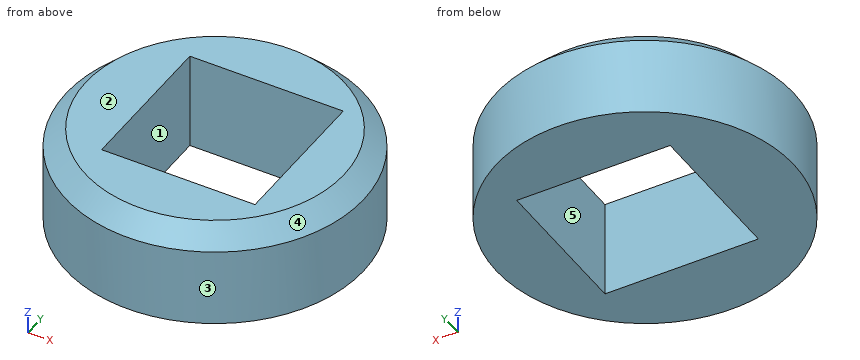
from build123d import *

# Parameters (mm, degrees)
F0_R     = 37.945444
F1_DEPTH = 25
F2_W     = 39.141135
F2_H     = 38.724022
F3_DEPTH = 25
F4_SIZE  = 5


with BuildPart() as f1:
    # F0 (on Top) → F1 (new body)
    with BuildSketch(Plane.XY):
        Circle(F0_R)
    extrude(amount=F1_DEPTH)

    # F2 (on face) → F3 (cut)
    with BuildSketch(Plane.XY.offset(25)):
        with Locations((1.78278, 0.198509)):
            Rectangle(F2_W, F2_H)
    extrude(amount=-F3_DEPTH, mode=Mode.SUBTRACT)

    # F4
    f4_edges = [f1.edges().sort_by_distance(p)[0] for p in [
        (-37.945444, 0, 25),
    ]]
    chamfer(f4_edges, length=F4_SIZE)


solid = f1.part
Could you check a few things on this model? Use its own coordinates, in mm. Face numbers are marked on the shaded views. A direction names the side the tool comes from. Give positions to 0.01 mm unless a question says otherwise; leave off trailing zeros. Order: outer loops, then holes, each group sorted by start corner. A loop starts at its lowest first (then second) coordinate and runs counter-clockwise, first axis right, second up. Notation, with made-up numbers: (29, -15) -> (81, -15) arc R18 cw to (81, -9) -> close; hole circle Ø1 at (7, -6). An arc over 180 degrees is marked (long way). Return JSON: item names as keys, results as strings.
1. Thinking about a two-plate mould opening in Y: for the marked faces 1, 2 and 3, which applies, pulls with the +Y half, pulls with the -Y half, needs draft (parallel to the pull), parting line crosses it, or undercut?
Answer list:
{"face 1": "undercut", "face 2": "needs draft", "face 3": "parting line crosses it"}
2. For pin 1 Ø7.5 at (y, z) = (2, 16.5) entering from +X; pin 2 Ø5 at (x, z) = (30, 20.5) entering from -Y; pin 3 Ø10 at (y, z) = (-22, 14) entering from -X; pin 4 Ø12.5 at (x, z) = (-1, 16) entering from -Y, each with a flat end and sliding along its axis, tell me the tip position at first contact or that it passes through.
Answer list:
{"pin 1": "stops at x = 37.95", "pin 2": "stops at y = -26.09", "pin 3": "stops at x = -33.92", "pin 4": "stops at y = -37.95"}
3. On a 3-axis mill with a long thin cutter (end or side, diameter ignored), from which of +Z, -Z, +X, -X, +Y, -Y can I reach the whole of each face in a straight line? I mean the marked faces 4 and 5. Say none if no direction works.
Answer list:
{"face 4": "+Z", "face 5": "+Z, -Z"}
4. I need wall thicknesses on line 1 (X direction, y = 0.5, z = 17.5); line 2 (X direction, y = -9, z = 3); line 3 (Y direction, x = 16, z = 9.5). Which ranges of each line are inside material? Lowest first, please. Write a range as from..to.
Answer list:
{"line 1": "x = -37.94..-17.79, 21.35..37.94", "line 2": "x = -36.86..-17.79, 21.35..36.86", "line 3": "y = -34.41..-19.16, 19.56..34.41"}
5. Imagine slicing it at B-B on y = 0. List the corners of the cut face in (x, z) for me.
Answer list:
{"outline": "(-37.95, 0) -> (-17.79, 0) -> (-17.79, 25) -> (-32.95, 25) -> (-37.95, 20) -> close; (21.35, 0) -> (37.95, 0) -> (37.95, 20) -> (32.95, 25) -> (21.35, 25) -> close"}
6. Imagine slicing it at A-A on x = 0. List the corners of the cut face in (y, z) for me.
Answer list:
{"outline": "(-37.95, 0) -> (-19.16, 0) -> (-19.16, 25) -> (-32.95, 25) -> (-37.95, 20) -> close; (19.56, 0) -> (37.95, 0) -> (37.95, 20) -> (32.95, 25) -> (19.56, 25) -> close"}
7. Imagine slicing it at C-C on z = 7.5. List the corners of the cut face in (x, y) for me.
Answer list:
{"outline": "circle Ø75.89 at (0, 0); hole (-17.79, -19.16) -> (21.35, -19.16) -> (21.35, 19.56) -> (-17.79, 19.56) -> close"}
